Verification items for the finished model (mm, model axes). A direction names the side the tool comes from. Round coordinates to 2 decimals unless told otherwise and drop trailing zeros. Write each loop counter-clockwise with the first axis right and the second up, starting at its lowest first coordinate (ties: lowest second). Pieces come first, ordered by that corner, then holes. Notation, with made-up numbers: M 47.5,42 L 52.5,42 A12 cw 52.5,54 Z; hole C 84,37 d6. An arc over 180 degrees is marked long. One line per item, written item: value. Start each with the question number.
from build123d import *

# Parameters (mm, degrees)
F1_DEPTH  = 48.26
F3_DEPTH  = 8.382
F5_DEPTH  = 8.382
F6_R      = 1.8288
F7_DEPTH  = 32.8422
F9_DEPTH  = 57.15
F10_W     = 2.286
F10_H     = 3.556
F11_DEPTH = 48.768
F12_R     = 2.286


with BuildPart() as f1:
    # F0 (on Top) → F1 (new body)
    with BuildSketch(Plane.XY):
        with BuildLine():
            ThreePointArc((-38.1, -38.1), (0, -50.8), (38.1, -38.1))
            Line((38.1, -38.1), (38.1, 38.1))
            ThreePointArc((38.1, 38.1), (0, 50.8), (-38.1, 38.1))
            Line((-38.1, 38.1), (-38.1, -38.1))
        make_face()
    extrude(amount=-F1_DEPTH)

    # F2 (on face) → F3 (join)
    with BuildSketch(Plane.XY):
        with BuildLine():
            Line((-34.925, 36.486888), (-34.925, -36.486888))
            ThreePointArc((-34.925, -36.486888), (0, -47.625), (34.925, -36.486888))
            Line((34.925, -36.486888), (34.925, 36.486888))
            ThreePointArc((34.925, 36.486888), (0, 47.625), (-34.925, 36.486888))
        make_face()
    extrude(amount=F3_DEPTH)

    # F4 (on face) → F5 (cut, through all)
    with BuildSketch(Plane.XY.offset(8.382)):
        with BuildLine():
            ThreePointArc((-26.67, -38.092896), (-25.275443, -32.88834), (-30.48, -31.493783))
            Line((-30.48, -31.493783), (-52.477045, -44.193783))
            ThreePointArc((-52.477045, -44.193783), (-53.871602, -49.39834), (-48.667045, -50.792896))
            Line((-48.667045, -50.792896), (-26.67, -38.092896))
        make_face()
        with BuildLine():
            ThreePointArc((30.48, -31.493783), (25.275443, -32.88834), (26.67, -38.092896))
            Line((26.67, -38.092896), (48.667045, -50.792896))
            ThreePointArc((48.667045, -50.792896), (53.871602, -49.39834), (52.477045, -44.193783))
            Line((52.477045, -44.193783), (30.48, -31.493783))
        make_face()
        with BuildLine():
            Line((-52.477045, 44.193783), (-30.48, 31.493783))
            ThreePointArc((-30.48, 31.493783), (-25.275443, 32.88834), (-26.67, 38.092896))
            Line((-26.67, 38.092896), (-48.667045, 50.792896))
            ThreePointArc((-48.667045, 50.792896), (-53.871602, 49.39834), (-52.477045, 44.193783))
        make_face()
        with BuildLine():
            ThreePointArc((26.67, 38.092896), (25.275443, 32.88834), (30.48, 31.493783))
            Line((30.48, 31.493783), (52.477045, 44.193783))
            ThreePointArc((52.477045, 44.193783), (53.871602, 49.39834), (48.667045, 50.792896))
            Line((48.667045, 50.792896), (26.67, 38.092896))
        make_face()
    extrude(amount=-F5_DEPTH, mode=Mode.SUBTRACT)

    # F6 (on face) → F7 (cut)
    with BuildSketch(Plane.XY):
        with Locations((28.575, -34.79334)):
            Circle(F6_R)
        with Locations((-28.575, -34.79334)):
            Circle(F6_R)
        with Locations((-28.575, 34.79334)):
            Circle(F6_R)
        with Locations((28.575, 34.79334)):
            Circle(F6_R)
    extrude(amount=-F7_DEPTH, mode=Mode.SUBTRACT)

    # F8 (on Top) → F9 (join)
    with BuildSketch(Plane.XY):
        with BuildLine():
            ThreePointArc((-12.7, 6.35), (0, -6.35), (12.7, 6.35))
            Line((12.7, 6.35), (12.7, 31.75))
            ThreePointArc((12.7, 31.75), (0, 44.45), (-12.7, 31.75))
            Line((-12.7, 31.75), (-12.7, 6.35))
        make_face()
    extrude(amount=F9_DEPTH)

    # F10 (on face) → F11 (join, through all)
    with BuildSketch(Plane.XY.offset(8.382)):
        with Locations((-13.843, 11.684)):
            Rectangle(F10_W, F10_H)
    extrude(amount=F11_DEPTH)

    # F12
    f12_edges = [f1.edges().sort_by_distance(p)[0] for p in [
        (12.7, 19.05, 57.15),
    ]]
    fillet(f12_edges, radius=F12_R)


solid = f1.part
1) Cross-section at A-A (x = 0). Record the boundary of the cut face in (y, z) (3 decimals), then the cut area to 3 significant figures.
2) Gauge pin test, flat ends, axial feed: pin 1 Ø9 at (y, z) = (-10.5, 5.5) entering from -X (3 decimals); pin 2 Ø1.8 at (x, y) = (-28, 35) entering from +Z; pin 3 Ø1 at (x, z) = (3.5, 18) entering from -Y. Record the tip position at first contact, or that the pin passes through.
3) Access from +Z, -Z, +X, -X, +Y, -Y to the whole of each face (thin tool, end or side, straight path). Record for faces 1 (the flat face through (34.925, 0, 4)), 2 (the cylindrical face through (-26.83, 35.34, -16.19)), 3 (the cylindrical face through (0.434, 47.623, 4.132)), 4 (the flat face through (-14, 9.906, 32)).
4) Mould release check, pull along Y, two halves, no side actions. Record for faces 5 (the flat face through (-28.149, 38.947, 4.25)), 6 (the flat face through (0, 19, 57.15)), 7 (the flat face through (32.734, -32.795, 4.25)): pulls with the +Y half, pulls with the -Y half, needs draft (parallel to the pull), parting line crosses it, or undercut.
5) Cross-section at D-D (y = -22). Record the boundary of the cut face in (x, z) (3 decimals).
6) Cross-section at C-C (z = -18.5). Record the boundary of the cut face in (x, y) (3 decimals).
7) Thickness scan on line 1 (Y direction, x = -28, z = -28.5); line 2 (Y direction, x = -11, z = 18); line 3 (Z direction, x = -25, y = -28). Record the ranges inside material, lowest first.
8) Cross-section at B-B (y = 16). Record the boundary of the cut face in (x, z) (3 decimals), then the cut area to 3 significant figures.
Results below:
1. outline: M -50.8,-48.26 L 50.8,-48.26 L 50.8,0 L 47.625,0 L 47.625,8.382 L 44.45,8.382 L 44.45,54.864 A2.286 ccw 42.164,57.15 L -4.064,57.15 A2.286 ccw -6.35,54.864 L -6.35,8.382 L -47.625,8.382 L -47.625,0 L -50.8,0 Z
1. area: 8,180 mm²
2. pin 1: stops at x = -34.925
2. pin 2: stops at z = -32.84
2. pin 3: stops at y = -5.99
3. face 1: +Z, +X, +Y, -Y
3. face 2: +Z
3. face 3: +Z, +Y
3. face 4: +Z, -X, -Y
4. face 5: undercut
4. face 6: needs draft
4. face 7: pulls with the -Y half
5. outline: M -38.1,-48.26 L 38.1,-48.26 L 38.1,0 L 34.925,0 L 34.925,8.382 L -34.925,8.382 L -34.925,0 L -38.1,0 Z
6. outline: M -38.1,-38.1 A63.5 ccw 38.1,-38.1 L 38.1,38.1 A63.5 ccw -38.1,38.1 Z; hole C -28.575,-34.793 d3.658; hole C -28.575,34.793 d3.658; hole C 28.575,-34.793 d3.658; hole C 28.575,34.793 d3.658
7. line 1: y = -44.29 to -36.53, -33.06 to 33.06, 36.53 to 44.29
7. line 2: y = 0 to 38.1
7. line 3: z = -48.26 to 8.38
8. outline: M -38.1,-48.26 L 38.1,-48.26 L 38.1,0 L 34.925,0 L 34.925,8.382 L 12.7,8.382 L 12.7,54.864 A2.286 ccw 10.414,57.15 L -10.414,57.15 A2.286 ccw -12.7,54.864 L -12.7,8.382 L -34.925,8.382 L -34.925,0 L -38.1,0 Z
8. area: 5,500 mm²
